Autodesk Inventor part; units mm, degrees
ref_plane "Work Plane1" through (52.918584, 12.839746, 0) normal (0.8660254, 0.5, 0) x (-0.5, 0.8660254, 0)
ref_plane "Work Plane2" through (53.588457, 10.339746, 0) normal (1, 0, 0) x (0, 1, 0)
ref_plane "YZ Plane" through (0, 0, 0) normal (1, 0, 0) x (0, 1, 0)
sketch "Sketch1" plane through (0, 0, 0) normal (0, 0, 1) x (1, 0, 0)
  line L0 (53.588457, 0) -> (0, 0)
  line L1 (0, 0) -> (60.328682, 34.830781)
  line L2 (43.588457, 0) -> (43.588457, 7.660254)
  line L3 (42.918584, 10.160254) -> (36.588457, 21.124356)
  line L4 (53.588457, 0) -> (53.588457, 10.339746)
  line L5 (52.918584, 12.839746) -> (45.248711, 26.124356)
  arc A0 (43.588457, 7.660254) -> (42.918584, 10.160254) centre (38.588457, 7.660254) ccw
  arc A1 (53.588457, 10.339746) -> (52.918584, 12.839746) centre (48.588457, 10.339746) ccw
  line L6 (45.248711, 26.124356) -> (36.588457, 21.124356)
  line L7 (45.248711, 26.124356) -> (52.918584, 12.839746)
  line L8 (36.588457, 21.124356) -> (42.918584, 10.160254)
  line L9 (43.588457, 0) -> (53.588457, 0)
  line L10 (53.588457, 0) -> (53.588457, 10.339746)
  line L11 (43.588457, 0) -> (53.588457, 0)
  line L12 (53.588457, 0) -> (53.588457, 10.339746)
  line L13 (52.918584, 12.839746) -> (45.248711, 26.124356)
  line L14 (45.248711, 26.124356) -> (36.588457, 21.124356)
  line L15 (36.588457, 21.124356) -> (42.918584, 10.160254)
  line L16 (43.588457, 7.660254) -> (43.588457, 0)
  point P0 (43.30127, 25)
  point P1 (43.588457, 9)
  dimension "d37" = 30
  dimension "d38" = 10
  dimension "d39" = 10
  dimension "d40" = 0
  dimension "d41" = 0
  dimension "d42" = 9
  dimension "d43" = 14
  dimension "d44" = 150
  dimension "d45" = 5
extrude "Extrusion1" add sketch "Sketch1" along normal blind 12 contours L0 L2 A0 L3 L1 L5 A1 L4
ref_plane "Work Plane1" through (52.918584, 12.839746, 0) normal (0.8660254, 0.5, 0) x (-0.5, 0.8660254, 0)
sketch "Sketch2" plane through (52.918584, 12.839746, 0) normal (0.8660254, 0.5, 0) x (-0.5, 0.8660254, 0)
  circle A0 centre (15.339746, 6) radius 6
  line L0 (15.339746, 0) -> (15.339746, 12)
  line L1 (0, 12) -> (15.339746, 12)
  dimension "d5" = 12
  dimension "d47" = 0
  dimension "d48" = 6
extrude "Extrusion2" add sketch "Sketch2" against normal blind 10
ref_plane "Work Plane2" through (53.588457, 10.339746, 0) normal (1, 0, 0) x (0, 1, 0)
sketch "Sketch3" plane through (53.588457, 10.339746, 0) normal (1, 0, 0) x (0, 1, 0)
  circle A0 centre (-10.339746, 6) radius 6
  line L0 (-10.339746, 0) -> (-10.339746, 12)
  line L1 (-10.339746, 0) -> (0, 0)
  point P0 (43.30127, 10)
  point P1 (10.78461, 12)
  dimension "d10" = 12
  dimension "d49" = 0
  dimension "d50" = 6
extrude "Extrusion3" add sketch "Sketch3" against normal blind 10
sketch "Sketch4" plane through (44.25833, 7.839746, 0) normal (-0.8660254, -0.5, 0) x (0.5, -0.8660254, 0)
  circle A0 centre (-15.339746, 6) radius 2.5
  circle A1 centre (-15.339746, 6) radius 6
  point P0 (-15.339746, 0)
  point P1 (-15.339746, 12)
  dimension "d15" = 5
extrude "Extrusion4" cut sketch "Sketch4" along normal through all both and the other way through all contours A0
sketch "Sketch5" plane through (43.588457, 10.339746, 0) normal (-1, 0, 0) x (0, 0, 1)
  circle A0 centre (6, -10.339746) radius 2.5
  arc A1 (0, -10.339746) -> (12, -10.339746) centre (6, -10.339746) ccw
  dimension "d18" = 5
extrude "Extrusion5" cut sketch "Sketch5" along normal through all both and the other way through all
sketch "Sketch6" plane through (52.918584, 12.839746, 0) normal (0.8660254, 0.5, 0) x (0.5, -0.8660254, 0)
  circle A0 centre (-15.339746, -6) radius 3.6
  circle A1 centre (-15.339746, -6) radius 2.5
  arc A2 (-15.339746, 0) -> (-15.339746, 0) centre (-15.339746, -6) ccw
  point P0 (0, -10)
  dimension "d21" = 5
  dimension "d22" = 7.2
extrude "Extrusion6" cut sketch "Sketch6" against normal blind 3 contours A0
sketch "Sketch7" plane through (44.25833, 7.839746, 0) normal (-0.8660254, -0.5, 0) x (0.5, -0.8660254, 0)
  circle A0 centre (-15.339746, 6) radius 3.6
  circle A1 centre (-15.339746, 6) radius 2.5
  arc A2 (-12.839746, 6) -> (-12.839746, 6) centre (-15.339746, 6) ccw
  point P0 (-15.339746, 0)
  dimension "d25" = 5
  dimension "d26" = 7.2
extrude "Extrusion7" cut sketch "Sketch7" along normal mid plane 6
sketch "Sketch8" plane through (43.588457, 10.339746, 0) normal (-1, 0, 0) x (0, 0, 1)
  circle A0 centre (6, -10.339746) radius 3.6
  circle A1 centre (6, -10.339746) radius 2.5
  arc A2 (8.5, -10.339746) -> (8.5, -10.339746) centre (6, -10.339746) ccw
  point P0 (0, -10.339746)
  dimension "d29" = 7.2
  dimension "d30" = 5
extrude "Extrusion8" cut sketch "Sketch8" along normal mid plane 6
sketch "Sketch9" plane through (53.588457, 10.339746, 0) normal (1, 0, 0) x (0, 0, -1)
  circle A0 centre (-6, -10.339746) radius 3.6
  circle A1 centre (-6, -10.339746) radius 2.5
  circle A2 centre (-6, -10.339746) radius 2.5
  point P0 (0, -10.339746)
  dimension "d33" = 5
  dimension "d34" = 7.2
extrude "Extrusion9" cut sketch "Sketch9" against normal blind 3
fillet "Fillet1" radius 2 16 edges at (42.2487, 31.3205, 6) (49.0836, 19.4821, 0) (53.4181, 11.6338, 0) (53.5885, 5.1699, 0) (53.5885, -6, 6) (53.5885, 5.1699, 12) (53.4181, 11.6338, 12) (49.0836, 19.4821, 12) (43.4181, 8.9543, 12) (43.5885, 3.8301, 12) (43.5885, -6, 6) (43.5885, 3.8301, 0) (43.4181, 8.9543, 0) (39.7535, 15.6423, 0) (33.5885, 26.3205, 6) (39.7535, 15.6423, 12)
equation "\"d38\" = d46"
equation "\"d39\" = d46"
equation "\"d3\" = width"
equation "\"d5\" = width"
equation "\"d48\" = 0.5 * width"
equation "\"d8\" = thickness"
equation "\"d10\" = width"
equation "\"d50\" = 0.5 * width"
equation "\"d13\" = thickness"
equation "\"thickness\" = 10"
equation "\"width\" = 12"
equation "\"d46\" = 10"
properties part number "Link2"
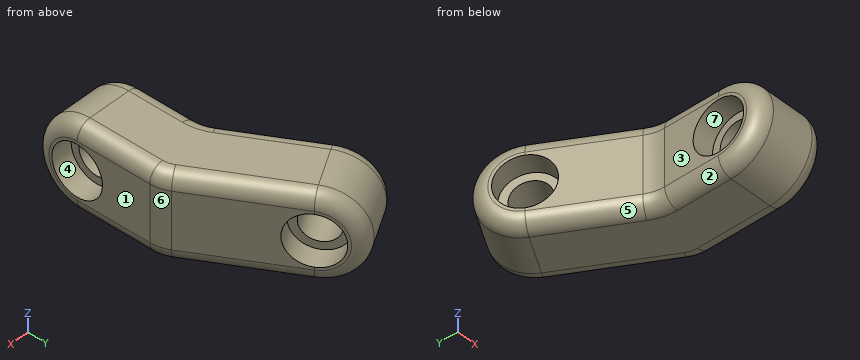
Work out the finished part from the listing and answer in its coordinate system (mm). Face numbers are marked on the shaded views. A direction names the side the tool comes from. Coordinates: 2 decimals unless noted, no trailing zeros. Order: outer loops, then holes, each group sorted by start corner. A loop starts at its lowest first (then second) coordinate and runs counter-clockwise, first axis right, second up. Notation, with made-up numbers: (70, 7.25) - (83, 7.25) arc R23 ccw to (83, 27.25) - close; hole circle Ø5 at (27, 27). An arc over 180 degrees is marked (long way). Answer as a JSON object with one key per item and string values.
1. Each of these flat-tipped pins is pushed along its axis until it touches: P1, Ø4, axis at y = 12, z = 7.5, coming from the -X side; P2, Ø6, axis at x = 49.5, z = 9.5, coming from the -Y side; P3, Ø1.5, axis at y = 20, z = 4, coming from the +X side. Where does it stop, or does it pass through?
Output values:
{"P1": "stops at x = 40.7", "P2": "stops at y = -5.98", "P3": "stops at x = 49.22"}
2. Find section B-B on z = 6. Count the separate pieces of the cut face and the enclosed holes in it, plus the area to 3 significant figures.
Output values:
{"separate pieces": "3", "enclosed holes": "0", "area": "247 mm²"}
3. The mould has two halves that part along Y. Classify the marked faces 5, 6 and 7: +Y half, -Y half, draft (parallel to the pull), parting line (faces both ways), or undercut.
Output values:
{"face 5": "-Y half", "face 6": "+Y half", "face 7": "undercut"}
4. Consider line 1 (X direction, y = 5, z = 3); line 2 (Y direction, x = 44.55, z = 6); line 3 (Y direction, x = 45.5, z = 6). Determine where each line is inside the solid, lowest interval first.
Output values:
{"line 1": "x = 43.59 to 53.59", "line 2": "y = -5.71 to -3.6, 3.6 to 21.56", "line 3": "y = -6 to -3.6, 3.6 to 22.11"}
5. Find section A-A on y = 4. Determine the outline of the cut face in (x, z), plus the area to 3 significant figures.
Output values:
{"outline": "(43.59, 2) arc R2 ccw to (45.59, 0) - (51.59, 0) arc R2 ccw to (53.59, 2) - (53.59, 10) arc R2 ccw to (51.59, 12) - (45.59, 12) arc R2 ccw to (43.59, 10) - close", "area": "117 mm²"}
6. A tool of negligible diameter and unlimited length cuts with its end or side. For the marked faces 1, 2, 3 and 4, from which of +Z, -Z, +X, -X, +Y, -Y can it reach the whole face along a straight path? Write none if from no direction.
Output values:
{"face 1": "+Z, -Z, +X, +Y, -Y", "face 2": "-Z, -X, -Y", "face 3": "+Z, -Z, -X, -Y", "face 4": "+X"}
